Source: CAD feature listing. Evaluate the final solid. Frame: model axes, mm. A direction names the side the tool comes from. Give positions to 0.01 mm unless a question says otherwise; leave off trailing zeros. Loops run counter-clockwise (first coordinate to the right, second up) from the corner with the lowest first, then second, coordinate; pieces in that order, holes last.
```python
from build123d import *

# Parameters (mm, degrees)
F0_W     = 127
F0_H     = 10.16
F0_H_2   = 10.284107
F1_DEPTH = 25.4
F2_W     = 4.572
F2_H     = 10.16
F3_DEPTH = 50.8
F4_W     = 4.572
F4_H     = 10.16
F5_DEPTH = 25.4


with BuildPart() as f1:
    # F0 (on Top) → F1 (new body)
    with BuildSketch(Plane.XY):
        Polygon((116.738255, 63.828293), (78.638255, 63.828293), (78.638255, 53.668293), (78.638255, -52.8876), (78.638255, -63.171707), (116.738255, -63.171707), align=None)
        with Locations((15.138255, 58.748293)):
            Rectangle(F0_W, F0_H)
        Polygon((-48.361745, 53.668293), (-48.361745, 63.828293), (-86.461745, 63.828293), (-86.461745, -63.171707), (-48.361745, -63.171707), (-48.361745, -52.8876), align=None)
        with Locations((15.138255, -58.029653)):
            Rectangle(F0_W, F0_H_2)
    extrude(amount=F1_DEPTH)

    # F2 (on Top) → F3 (join)
    with BuildSketch(Plane.XY):
        with Locations((-50.779041, -0.207529)):
            Rectangle(F2_W, F2_H)
    extrude(amount=F3_DEPTH)

    # F4 (on face) → F5 (join)
    with BuildSketch(Plane.XY.offset(25.4)):
        with Locations((80.924255, 1.138359)):
            Rectangle(F4_W, F4_H)
    extrude(amount=F5_DEPTH)


solid = f1.part
```
(1) Mould query, pull axis Y, two halves, no side actions, for faces 1 (the flat face through (116.738, -1, 13)), 2 (the flat face through (81, 6.218, 38)), 3 (the flat face through (-48.362, 0, 13)). Classes: pulls with the +Y half, pulls with the -Y half, needs draft (parallel to the pull), parting line crosses it, or undercut.
A:
face 1: needs draft
face 2: pulls with the +Y half
face 3: undercut
(2) Section D-D, the plane y = -55. Return the cut outline in (x, z), then the cut area to 3 significant figures.
A:
outline: (-86.46, 0) - (116.74, 0) - (116.74, 25.4) - (-86.46, 25.4) - close
area: 5,160 mm2
(3) Ray query, line 1 along X through (y, z) = (8.5, 23); line 2 along Y through (x, z) = (55.5, 7); line 3 along Z through (x, y) = (32, 56). Return the intervals inside material, ascending.
A:
line 1: x = -86.46 to -48.36, 78.64 to 116.74
line 2: y = -63.17 to -52.89, 53.67 to 63.83
line 3: z = 0 to 25.4
(4) Section A-A, the plane y = -23.5. Return the cut outline in (x, z), then the cut area to 3 significant figures.
A:
outline: (-86.46, 0) - (-48.36, 0) - (-48.36, 25.4) - (-86.46, 25.4) - close; (78.64, 0) - (116.74, 0) - (116.74, 25.4) - (78.64, 25.4) - close
area: 1,940 mm2
(5) Reachability of faces 4 (the flat face through (-86.462, 1, 13)), 5 (the flat face through (81, -3.942, 38)), 6 (the flat face through (14, -52.888, 13)), 7 (the flat face through (-51, 4.872, 38)), 8 (the flat face through (-53.065, 0, 38)) from +Z, -Z, +X, -X, +Y, -Y: full face, straight path, thin tool, end or side. Return the list, or none.
A:
face 4: +Z, -Z, -X, +Y, -Y
face 5: +Z, +X, -Y
face 6: +Z, -Z
face 7: +Z, -X, +Y
face 8: +Z, -X, +Y, -Y
(6) Section C-C, the plane x = 26.5. Return the cut outline in (y, z).
A:
outline: (-63.17, 0) - (-52.89, 0) - (-52.89, 25.4) - (-63.17, 25.4) - close; (53.67, 0) - (63.83, 0) - (63.83, 25.4) - (53.67, 25.4) - close
(7) First-contact query: pin 1 (11 mm diameter, centred on y = 3.5, z = 37.5, fed in from +X); pin 2 (1.4 mm diameter, centred on x = -50, z = 42.5, fed in from +Y); pin 3 (5 mm diameter, centred on x = 81, z = 38, fed in from -Y). Flat tips, straight axial feed; report the tip coordinate or a pass-through.
A:
pin 1: stops at x = 83.21
pin 2: stops at y = 4.87
pin 3: stops at y = -3.94
(8) Section B-B, the plane z = 21. Return the cut outline in (x, y), then the cut area to 3 significant figures.
A:
outline: (-86.46, -63.17) - (116.74, -63.17) - (116.74, 63.83) - (-86.46, 63.83) - close; hole (-48.36, -52.89) - (78.64, -52.89) - (78.64, 53.67) - (-48.36, 53.67) - close
area: 12,300 mm2
